```python
from build123d import *

# Parameters (mm, degrees)
SKETCH2_R           = 21
BOSS_EXTRUDE1_DEPTH = 3.5
CUT_EXTRUDE1_DEPTH  = 2.25
SKETCH4_R           = 5.5
SKETCH4_R_2         = 1.143
SKETCH4_R_3         = 1.5875
CUT_EXTRUDE2_DEPTH  = 4.5
CUT_EXTRUDE4_DEPTH  = 2.25
SKETCH6_W           = 2.148549125
SKETCH6_H           = 1


with BuildPart() as part:
    # Sketch2 → Boss-Extrude1 (new body)
    with BuildSketch(Plane(origin=(0, 0, 0), x_dir=(1, 0, 0), z_dir=(0, 1, 0))):
        Circle(SKETCH2_R)
    extrude(amount=BOSS_EXTRUDE1_DEPTH)

    # Sketch1 → Cut-Extrude1 (cut)
    with BuildSketch(Plane(origin=(0, 0, 0), x_dir=(1, 0, 0), z_dir=(0, 1, 0))):
        with BuildLine():
            Line((-2.382460832, -18.999213313), (-4.483221098, -6.564797513))
            ThreePointArc((-4.483221098, -6.564797513), (-5.191745443, -5.191745443), (-6.564797513, -4.483221098))
            Line((-6.564797513, -4.483221098), (-18.999213313, -2.382460832))
            ThreePointArc((-18.999213313, -2.382460832), (-20, 0), (-18.999213313, 2.382460832))
            Line((-18.999213313, 2.382460832), (-6.564797513, 4.483221098))
            ThreePointArc((-6.564797513, 4.483221098), (-5.191745443, 5.191745443), (-4.483221098, 6.564797513))
            Line((-4.483221098, 6.564797513), (-2.382460832, 18.999213313))
            ThreePointArc((-2.382460832, 18.999213313), (0, 20), (2.382460832, 18.999213313))
            Line((2.382460832, 18.999213313), (4.483221098, 6.564797513))
            ThreePointArc((4.483221098, 6.564797513), (5.191745443, 5.191745443), (6.564797513, 4.483221098))
            Line((6.564797513, 4.483221098), (18.999213313, 2.382460832))
            ThreePointArc((18.999213313, 2.382460832), (20, 0), (18.999213313, -2.382460832))
            Line((18.999213313, -2.382460832), (6.564797513, -4.483221098))
            ThreePointArc((6.564797513, -4.483221098), (5.191745443, -5.191745443), (4.483221098, -6.564797513))
            Line((4.483221098, -6.564797513), (2.382460832, -18.999213313))
            ThreePointArc((2.382460832, -18.999213313), (0, -20), (-2.382460832, -18.999213313))
        make_face()
    extrude(amount=CUT_EXTRUDE1_DEPTH, mode=Mode.SUBTRACT)

    # Sketch4 → Cut-Extrude2 (cut, through all)
    with BuildSketch(Plane(origin=(0, 3.5, 0), x_dir=(1, 0, 0), z_dir=(0, 1, 0))):
        Circle(SKETCH4_R)
        with Locations((7.445, 0)):
            Circle(SKETCH4_R_2)
        with Locations((10.54, 0)):
            Circle(SKETCH4_R_2)
        with Locations((13.46, 0)):
            Circle(SKETCH4_R_2)
        with Locations((16.51, 0)):
            Circle(SKETCH4_R_2)
        with Locations((10, 10)):
            Circle(SKETCH4_R_3)
        with Locations((0, -7.445)):
            Circle(SKETCH4_R_2)
        with Locations((0, -10.54)):
            Circle(SKETCH4_R_2)
        with Locations((0, -13.46)):
            Circle(SKETCH4_R_2)
        with Locations((0, -16.51)):
            Circle(SKETCH4_R_2)
        with Locations((10, -10)):
            Circle(SKETCH4_R_3)
        with Locations((-7.445, 0)):
            Circle(SKETCH4_R_2)
        with Locations((-10.54, 0)):
            Circle(SKETCH4_R_2)
        with Locations((-13.46, 0)):
            Circle(SKETCH4_R_2)
        with Locations((-16.51, 0)):
            Circle(SKETCH4_R_2)
        with Locations((-10, -10)):
            Circle(SKETCH4_R_3)
        with Locations((0, 7.445)):
            Circle(SKETCH4_R_2)
        with Locations((0, 10.54)):
            Circle(SKETCH4_R_2)
        with Locations((0, 13.46)):
            Circle(SKETCH4_R_2)
        with Locations((0, 16.51)):
            Circle(SKETCH4_R_2)
        with Locations((-10, 10)):
            Circle(SKETCH4_R_3)
    extrude(amount=-CUT_EXTRUDE2_DEPTH, mode=Mode.SUBTRACT)

    # Sketch5 → Cut-Extrude4 (cut)
    with BuildSketch(Plane(origin=(0, 3.5, 0), x_dir=(1, 0, 0), z_dir=(0, 1, 0))):
        Polygon((11.055981704, -13.940977371), (13.940977371, -11.055981704), (12.884995667, -7.115004333), (8.944018296, -6.059022629), (6.059022629, -8.944018296), (7.115004333, -12.884995667), align=None)
        Polygon((-8.944018296, 6.059022629), (-6.059022629, 8.944018296), (-7.115004333, 12.884995667), (-11.055981704, 13.940977371), (-13.940977371, 11.055981704), (-12.884995667, 7.115004333), align=None)
        Polygon((12.884995667, 7.115004333), (13.940977371, 11.055981704), (11.055981704, 13.940977371), (7.115004333, 12.884995667), (6.059022629, 8.944018296), (8.944018296, 6.059022629), align=None)
        Polygon((-7.115004333, -12.884995667), (-6.059022629, -8.944018296), (-8.944018296, -6.059022629), (-12.884995667, -7.115004333), (-13.940977371, -11.055981704), (-11.055981704, -13.940977371), align=None)
    extrude(amount=-CUT_EXTRUDE4_DEPTH, mode=Mode.SUBTRACT)

    # Sketch6 → Revolve1 (revolve)
    with BuildSketch(Plane.XY):
        with Locations((-21.425725437, 3)):
            Rectangle(SKETCH6_W, SKETCH6_H)
    revolve(axis=Axis((0, 0, 0), (0, 1, 0)))


solid = part.part
```
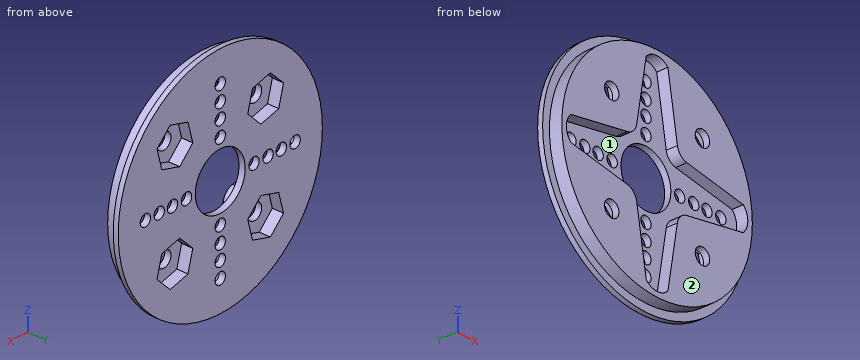
For this review, take the finished solid that the model builds, in its own axes (mm). Face numbers are marked on the shaded views. Coordinates: 2 decimals unless noted, no trailing zeros. Write each loop counter-clockwise with the first axis right and the second up, starting at its lowest first coordinate (ties: lowest second). Pieces come first, ordered by that corner, then holes. Notation, with made-up numbers: (8, 60) -> (19, 60) arc R24 ccw to (19, 75) -> close; hole circle Ø3 at (-26, 3). An arc over 180 degrees is marked (long way). Put each result on its own line as item: value.
Q1. Take a section at D-D, the plane x = 16.51. State the section outline as (y, z) points.
From the geometry:
outline: (0, -12.98) -> (2.5, -12.98) -> (2.5, -15.29) -> (3.5, -15.29) -> (3.5, -1.14) -> (2.25, -1.14) -> (2.25, -2.8) -> (0, -2.8) -> close; (0, 2.8) -> (2.25, 2.8) -> (2.25, 1.14) -> (3.5, 1.14) -> (3.5, 15.29) -> (2.5, 15.29) -> (2.5, 12.98) -> (0, 12.98) -> close
Q2. Wall thickness on L1, parallel to Z at x = 7.5, y = 3.25; L2, parallel to Y at x = 6, z = -3; L3, parallel to Z at x = -10.5, y = 2.6: over which ranges is each line inside the solid? List them lowest first.
From the geometry:
L1: z = -21.21 to -12.99, -7.5 to -1.14, 1.14 to 7.5, 12.99 to 21.21
L2: y = 2.25 to 3.5
L3: z = -19.9 to -13.79, -6.48 to -1.14, 1.14 to 6.48, 13.79 to 19.9
Q3. Clearance check with flat-ended pins moving along their axes: pin 1 Ø5 at (x, z) = (-10, 10) entering from +Y; pin 2 Ø3.5 at (x, z) = (0, -13.46) entering from -Y. State where each tip first meets the part, or that it passes through.
From the geometry:
pin 1: stops at y = 1.25
pin 2: stops at y = 2.25
Q4. The part is to be moulded in two halves that separate along Z. For the marked faces 1 and 2, say which applies: +Z half, -Z half, draft (parallel to the pull), parting line (faces both ways), or undercut.
From the geometry:
face 1: undercut
face 2: draft
Q5. Take a section at A-A, the plane y = 0.65. State the section outline as (x, z) points (1 decimal).
From the geometry:
outline: circle Ø42 at (0, 0); hole (-19, -2.4) -> (-6.6, -4.5) arc R2.5 cw to (-4.5, -6.6) -> (-2.4, -19) arc R3.3 ccw to (2.4, -19) -> (4.5, -6.6) arc R2.5 cw to (6.6, -4.5) -> (19, -2.4) arc R3.3 ccw to (19, 2.4) -> (6.6, 4.5) arc R2.5 cw to (4.5, 6.6) -> (2.4, 19) arc R3.3 ccw to (-2.4, 19) -> (-4.5, 6.6) arc R2.5 cw to (-6.6, 4.5) -> (-19, 2.4) arc R3.3 ccw to start; hole circle Ø3.2 at (-10, -10); hole circle Ø3.2 at (-10, 10); hole circle Ø3.2 at (10, -10); hole circle Ø3.2 at (10, 10)
Q6. Take a section at C-C, the plane z = -16.51. State the section outline as (x, y) points, then the cut area to 3 significant figures.
From the geometry:
outline: (-15.29, 2.5) -> (-12.98, 2.5) -> (-12.98, 0) -> (-2.8, 0) -> (-2.8, 2.25) -> (-1.14, 2.25) -> (-1.14, 3.5) -> (-15.29, 3.5) -> close; (1.14, 2.25) -> (2.8, 2.25) -> (2.8, 0) -> (12.98, 0) -> (12.98, 2.5) -> (15.29, 2.5) -> (15.29, 3.5) -> (1.14, 3.5) -> close
area: 80.0 mm2
Q7. Take a section at B-B, the plane x = -10.54. Count the separate pieces of the cut face and the enclosed holes in it, then the cut area to 3 significant figures.
From the geometry:
separate pieces: 4
enclosed holes: 0
area: 70.2 mm2
